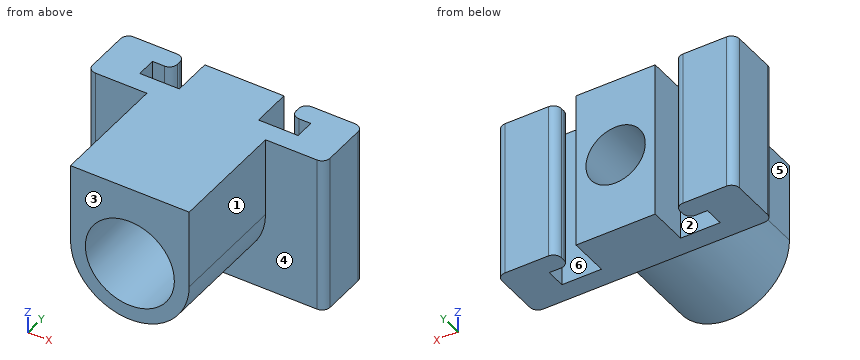
```python
from build123d import *

# Parameters (mm, degrees)
SKETCH1_W           = 38.1
SKETCH1_H           = 25.4
BOSS_EXTRUDE1_DEPTH = 9.525
CUT_EXTRUDE1_REACH  = 35.148
BOSS_EXTRUDE2_DEPTH = 19.05
CUT_EXTRUDE3_REACH  = 38.616
SKETCH5_R           = 4.7625
SKETCH4_R           = 7.14375
CUT_EXTRUDE2_DEPTH  = 19.05
FILLET2_R           = 1.27


with BuildPart() as part:
    # Sketch1 → Boss-Extrude1 (new body)
    with BuildSketch(Plane(origin=(0, 0, 0), x_dir=(1, 0, 0), z_dir=(0, 1, 0))):
        Rectangle(SKETCH1_W, SKETCH1_H)
    extrude(amount=BOSS_EXTRUDE1_DEPTH)

    # Sketch2 → Cut-Extrude1 (cut, up to next)
    with BuildSketch(Plane(origin=(0, 0, -12.7), x_dir=(-1, 0, 0), z_dir=(0, 0, -1)), mode=Mode.PRIVATE) as cut_extrude1_sk1:
        Polygon((-9.525, 9.525), (-9.525, 6.35), (-12.7, 6.35), (-12.7, 3.175), (-6.35, 3.175), (-6.35, 9.525), align=None)
    cut_extrude1_tool1 = extrude(cut_extrude1_sk1.sketch, amount=-CUT_EXTRUDE1_REACH, mode=Mode.PRIVATE) & part.part
    cut_extrude1 = cut_extrude1_tool1.solids().sort_by_distance((8.995833, 5.820833, -12.7))[0]
    add(cut_extrude1, mode=Mode.SUBTRACT)

    # Mirror1: Cut-Extrude1 across plane
    add(cut_extrude1.mirror(Plane(origin=(0, 0, 0), x_dir=(0, 0, 1), z_dir=(1, 0, 0))), mode=Mode.SUBTRACT)

    # Sketch3 → Boss-Extrude2 (add)
    with BuildSketch(Plane.XZ):
        with BuildLine():
            Line((9.525, 0), (9.525, 12.7))
            Line((9.525, 12.7), (-9.525, 12.7))
            Line((-9.525, 12.7), (-9.525, 0))
            ThreePointArc((-9.525, 0), (0, -9.525), (9.525, 0))
        make_face()
    extrude(amount=BOSS_EXTRUDE2_DEPTH)

    # Sketch5 → Cut-Extrude3 (cut, up to next)
    with BuildSketch(Plane(origin=(0, -19.05, 0), x_dir=(-1, 0, 0), z_dir=(0, -1, 0)), mode=Mode.PRIVATE) as cut_extrude3_sk1:
        with Locations(Location((0, 0, 0), (0, 0, 90))):
            Circle(SKETCH5_R)
    cut_extrude3_tool1 = extrude(cut_extrude3_sk1.sketch, amount=-CUT_EXTRUDE3_REACH, mode=Mode.PRIVATE) & part.part
    add(cut_extrude3_tool1.solids().sort_by_distance((0, -19.05, 0))[0], mode=Mode.SUBTRACT)

    # Sketch4 → Cut-Extrude2 (cut)
    with BuildSketch(Plane.XZ.offset(19.05)):
        with Locations(Location((0, 0, 0), (0, 0, 270))):
            Circle(SKETCH4_R)
    extrude(amount=-CUT_EXTRUDE2_DEPTH, mode=Mode.SUBTRACT)

    # Fillet2
    fillet2_edges = [part.edges().sort_by_distance(p)[0] for p in [
        (19.05, 0, 0),
        (-19.05, 0, 0),
        (-19.05, 9.525, 0),
        (19.05, 9.525, 0),
        (9.525, 6.35, 0),
        (9.525, 9.525, 0),
        (-9.525, 6.35, 0),
        (-9.525, 9.525, 0),
    ]]
    fillet(fillet2_edges, radius=FILLET2_R)


solid = part.part
```
Geometry check sheet. Reference: the model listing, model coordinates, mm. Face numbers are marked on the shaded views. A direction names the side the tool comes from. Coordinates: 2 decimals unless noted, no trailing zeros. Order: outer loops, then holes, each group sorted by start corner. A loop starts at its lowest first (then second) coordinate and runs counter-clockwise, first axis right, second up. Notation, with made-up numbers: (81.5, -22) - (90.5, -22) arc R22 cw to (90.5, 1) - close; hole circle Ø1 at (30.25, 53.25). An arc over 180 degrees is marked (long way). Answer in a Markdown table with one row per item. Add a question column.
1. Material ranges on L1, parallel to X at y = 5.75, z = -10; L2, parallel to X at y = 4.5, z = 0; L3, parallel to Y at x = -12, z = 10.5 (3 decimals), recorded low to high. Write a range as [from, to].
2. Section check B-B (y = 7). Give the number of separate pieces and of enclosed holes in the cut face, plus the area to 3 significant figures.
3. Access from +Z, -Z, +X, -X, +Y, -Y to the whole of each face (thin tool, end or side, straight path). Record for the marked faces 4, 5 and 6.
4. Gauge pin test, flat ends, axial feed: pin 1 Ø1.5 at (y, z) = (-10, 5) entering from -X (3 decimals); pin 2 Ø1 at (x, z) = (12, -2) entering from -Y; pin 3 Ø6.5 at (y, z) = (-10, 7) entering from +X (3 decimals). Record the tip position at first contact, or that the pin passes through.
5. Section check C-C (z = 11.25). Enter the section's corners in (x, y) (3 decimals), plus the area to 3 significant figures.
6. Draft check along X on the marked faces 1, 2 and 3. Enter one of: +X half, -X half, draft (parallel to the pull), parting line (faces both ways), or undercut.
Data:
| question | item | result |
|---|---|---|
| 1 | L1 | x = [-19.05, -12.7], [-6.35, 6.35], [12.7, 19.05] |
| 1 | L2 | x = [-19.05, -12.7], [-6.35, -4.76], [4.76, 6.35], [12.7, 19.05] |
| 1 | L3 | y = [0, 3.175], [6.35, 9.525] |
| 2 | separate pieces | 3 |
| 2 | enclosed holes | 1 |
| 2 | area | 727 mm² |
| 3 | face 4 | -Z, -Y |
| 3 | face 5 | +Z, -Z, -X, -Y |
| 3 | face 6 | +Z, -Z |
| 4 | pin 1 | stops at x = -9.525 |
| 4 | pin 2 | stops at y = 0 |
| 4 | pin 3 | stops at x = 9.525 |
| 5 | outline | (-19.05, 1.27) arc R1.27 ccw to (-17.78, 0) - (-9.525, 0) - (-9.525, -19.05) - (9.525, -19.05) - (9.525, 0) - (17.78, 0) arc R1.27 ccw to (19.05, 1.27) - (19.05, 8.255) arc R1.27 ccw to (17.78, 9.525) - (10.795, 9.525) arc R1.27 ccw to (9.525, 8.255) - (9.525, 7.62) arc R1.27 ccw to (10.795, 6.35) - (12.7, 6.35) - (12.7, 3.175) - (6.35, 3.175) - (6.35, 9.525) - (-6.35, 9.525) - (-6.35, 3.175) - (-12.7, 3.175) - (-12.7, 6.35) - (-10.795, 6.35) arc R1.27 ccw to (-9.525, 7.62) - (-9.525, 8.255) arc R1.27 ccw to (-10.795, 9.525) - (-17.78, 9.525) arc R1.27 ccw to (-19.05, 8.255) - close |
| 5 | area | 663 mm² |
| 6 | face 1 | +X half |
| 6 | face 2 | undercut |
| 6 | face 3 | draft |
